Autodesk Inventor part; units mm, degrees
ref_plane "XY Plane" through (0, 0, 0) normal (0, 0, 1) x (1, 0, 0)
sketch "Sketch1" plane through (0, 0, 0) normal (0, 0, 1) x (1, 0, 0)
  circle A0 centre (0, 0) radius 1
  circle A1 centre (0, 0) radius 4
extrude "Extrusion1" add sketch "Sketch1" along normal blind 13
sketch "Sketch2" plane through (0, 0, 13) normal (0, 0, 1) x (1, 0, 0)
  circle A0 centre (0, 0) radius 1
  circle A1 centre (0, 0) radius 4
  circle A2 centre (0, 0) radius 2
  dimension "d5" = 4
extrude "Extrusion2" add sketch "Sketch2" along normal blind 1.5 contours A2
sketch "Sketch3" plane through (0, 0, 0) normal (0, 0, -1) x (-1, 0, 0)
  circle A0 centre (0, 0) radius 1
  circle A1 centre (0, 0) radius 4
  circle A2 centre (0, 0) radius 1.05
  dimension "d8" = 2.1
extrude "Extrusion3" cut sketch "Sketch3" against normal blind 20 contours A2
sketch "Sketch4" plane through (0, 0, 0) normal (0, 0, -1) x (-1, 0, 0)
  circle A0 centre (0, 0) radius 1.05
  circle A1 centre (0, 0) radius 4
extrude "Extrusion4" add sketch "Sketch4" along normal blind 0.5
sketch "Sketch5" plane through (0, 0, -0.5) normal (0, 0, -1) x (-1, 0, 0)
  circle A0 centre (0, 0) radius 1.05
  circle A1 centre (0, 0) radius 4
extrude "Extrusion5" add sketch "Sketch5" along normal blind 0.5
sketch "Sketch6" plane through (0, 0, -1) normal (0, 0, -1) x (-1, 0, 0)
  circle A0 centre (0, 0) radius 1.05
  circle A1 centre (0, 0) radius 4
extrude "Extrusion6" cut sketch "Sketch6" against normal blind 1
chamfer "Chamfer2" distance 0.2 angle 45 1 edges at (1.05, 0, 0)
sketch "Sketch7" plane through (0, 0, 14.5) normal (0, 0, 1) x (1, 0, 0)
  circle A0 centre (0, 0) radius 2
  circle A1 centre (0, 0) radius 1.1
  dimension "d20" = 2.2
extrude "Extrusion7" cut sketch "Sketch7" against normal blind 30 contours A1
fillet "Fillet1" radius 0.3 1 edges at (-2, 0, 13)
chamfer "Chamfer3" distance 0.4 angle 45 1 edges at (-1.1, 0, 14.5)
properties material "PBT Plastic"
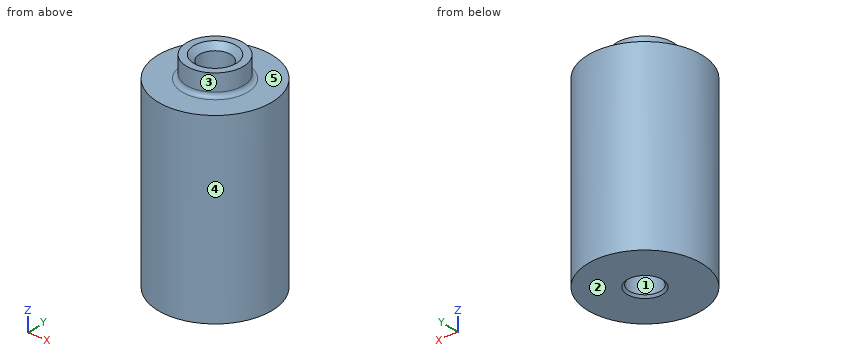
Model file for the job. Use its own axes, mm. Face numbers are marked on the shaded views. A direction names the side the tool comes from. Coordinates: 2 decimals unless noted, no trailing zeros. Loops run counter-clockwise (first coordinate to the right, second up) from the corner with the lowest first, then second, coordinate; pieces in that order, holes last. Notation, with made-up numbers: (-35, -17) -> (-15, -17) arc R21 cw to (-15, 9) -> close; hole circle Ø8 at (2.5, -8). An arc over 180 degrees is marked (long way). Use one line per item in the form item = value. Start each with the question number.
(1) Tool access for the marked faces 4 and 5: list every direction of +Z, -Z, +X, -X, +Y, -Y with a clear straight run to the whole face (end or side of a thin tool).
(2) Cut at D-D on x = 3.75. Give the cut face in (y, z), and give its area (3 significant figures).
(3) Probe probe 1 along Y at (x, z) = (0, 9.75); probe 2 along Z at (x, y) = (3.5, -1); probe 3 along X at (y, z) = (0.5, 3.25). List the from-to ranges inside material, lowest first. Write a range as from..to.
(4) Cut at A-A on y = 0. Give the cut face in (x, z).
(5) Cut at C-C on z = 6.75. Give the cut face in (x, y).
(6) Pull direction X, two halves, no side cores. Call the marked faces 1, 2 and 3: pulls with the +X half, pulls with the -X half, needs draft (parallel to the pull), parting line crosses it, or undercut.
(7) Flat gauge pins, fed straight in: pin 1 (1 mm diameter, centred on y = 2.5, z = 3, fed in from +X); pin 2 (1 mm diameter, centred on x = 1.5, z = 4, fed in from -Y); pin 3 (1 mm diameter, centred on y = -1, z = 2, fed in from -X). Where does each tip first touch, or does it go through?
Values:
q1.face_4 = +Z, -Z
q1.face_5 = +Z
q2.outline = (-1.39, 0) -> (1.39, 0) -> (1.39, 13) -> (-1.39, 13) -> close
q2.area = 36.2 mm2
q3.probe_1 = -4..-1.1, 1.1..4
q3.probe_2 = 0..13
q3.probe_3 = -3.97..-0.98, 0.98..3.97
q4.outline = (-4, 0) -> (-1.25, 0) -> (-1.1, 0.15) -> (-1.1, 14.1) -> (-1.5, 14.5) -> (-2, 14.5) -> (-2, 13.3) arc R0.3 cw to (-2.3, 13) -> (-4, 13) -> close; (1.1, 0.15) -> (1.25, 0) -> (4, 0) -> (4, 13) -> (2.3, 13) arc R0.3 cw to (2, 13.3) -> (2, 14.5) -> (1.5, 14.5) -> (1.1, 14.1) -> close
q5.outline = circle Ø8 at (0, 0); hole circle Ø2.2 at (0, 0)
q6.face_1 = undercut
q6.face_2 = needs draft
q6.face_3 = parting line crosses it
q7.pin_1 = 3.46
q7.pin_2 = -3.87
q7.pin_3 = -3.97
